Design review of the part built by this model. Coordinates are the model's own, in mm. Face numbers are marked on the shaded views. A direction names the side the tool comes from. Give positions to 0.01 mm unless a question says otherwise; leave off trailing zeros. Loops run counter-clockwise (first coordinate to the right, second up) from the corner with the lowest first, then second, coordinate; pieces in that order, holes last. Notation, with made-up numbers: M 16,40.5 L 66,40.5 A7 cw 66,53.5 Z; hole C 21.5,7.25 d2. An arc over 180 degrees is marked long. Answer as CSV lines item,"result".
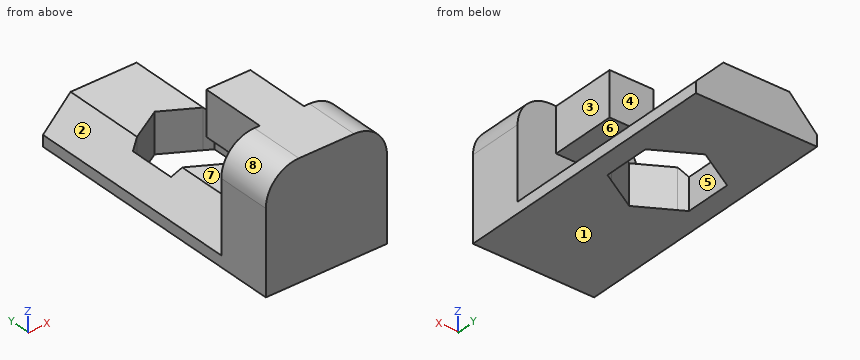
```python
from build123d import *

# Parameters (mm, degrees)
F1_DEPTH = 20
F3_DEPTH = 3.6
F4_W     = 11
F4_H     = 5
F5_DEPTH = 10.5
F6_W     = 4
F6_H     = 4
F7_DEPTH = 6
F8_R     = 3


with BuildPart() as f1:
    # F0 (on Front) → F1 (new body)
    with BuildSketch(Plane.XZ):
        Polygon((-5.5, 0), (5.5, 0), (5.5, 1), (3, 3.6), (0, 3.6), (-3, 3.6), (-5.5, 1), align=None)
    extrude(amount=F1_DEPTH)

    # F2 (on face) → F3 (cut, through all)
    with BuildSketch(Plane.XY.offset(3.6)):
        Polygon((3, -7.459659), (0, -5.727608), (-3, -7.459659), (-3, -12.540341), (0, -14.272392), (3, -12.540341), align=None)
        Polygon((3.7, -7.863804), (3, -7.459659), (3, -12.540341), (3.7, -12.136196), align=None)
        Polygon((-3, -12.540341), (-3, -7.459659), (-3.7, -7.863804), (-3.7, -12.136196), align=None)
    extrude(amount=-F3_DEPTH, mode=Mode.SUBTRACT)

    # F4 (on face) → F5 (join)
    with BuildSketch(Plane(origin=(0, 0, 0), x_dir=(1, 0, 0), z_dir=(0, 0, -1))):
        with Locations((0, 22.5)):
            Rectangle(F4_W, F4_H)
    extrude(amount=-F5_DEPTH)

    # F6 (on face) → F7 (join)
    with BuildSketch(Plane(origin=(0, -20, 0), x_dir=(-1, 0, 0), z_dir=(0, 1, 0))):
        with Locations((0, 8.5)):
            Rectangle(F6_W, F6_H)
    extrude(amount=F7_DEPTH)

    # F8
    f8_edges = [f1.edges().sort_by_distance(p)[0] for p in [
        (-5.5, -22.5, 10.5),
        (5.5, -22.5, 10.5),
    ]]
    fillet(f8_edges, radius=F8_R)


solid = f1.part
```
1. We need section B-B, the plane x = 2.75. Write out the cut boundary in (y, z).
Answer block:
outline,"M -25,0 L -12.68,0 L -12.68,3.6 L -20,3.6 L -20,10.49 L -25,10.49 Z; M -7.32,0 L 0,0 L 0,3.6 L -7.32,3.6 Z"
2. The part is to be moulded in two halves that separate along Z. For the marked faces 5, 6, 7 and 8, say which applies: pulls with the +Z half, pulls with the -Z half, needs draft (parallel to the pull), parting line crosses it, or undercut.
Answer block:
face 5,"needs draft"
face 6,"undercut"
face 7,"undercut"
face 8,"pulls with the +Z half"
3. We need section A-A, the plane y = -16.75. Write out the cut boundary in (x, z).
Answer block:
outline,"M -5.5,0 L 5.5,0 L 5.5,1 L 3,3.6 L -3,3.6 L -5.5,1 Z; M -2,6.5 L 2,6.5 L 2,10.5 L -2,10.5 Z"
4. For P1, Ø1.4, axis at y = -10.5, z = 1.5, coming from the +X side; P2, Ø5, axis at x = -2, z = 8, coming from the +Y side; P3, Ø3, axis at x = -1, y = -2, coming from the +Z side; P4, Ø3, axis at y = -16, z = 9, coming from the +X side, all flat-tipped, find the tip position at first contact; note any pin that passes through.
Answer block:
P1,"x = 5.5"
P2,"y = -14"
P3,"z = 3.6"
P4,"x = 2"
5. To check wall thickness, follow L1, parallel to Z at x = -1, y = -15; L2, parallel to Y at x = -2.5, z = 9.25; L3, parallel to X at y = -16.5, z = 7.5. State the ranges of each line that lie inside material, in increasing order. Write a range as [from, to].
Answer block:
L1,"[0, 3.6], [6.5, 10.5]"
L2,"[-25, -20]"
L3,"[-2, 2]"
6. We need section C-C, the plane z = 7. Write out the cut boundary in (x, y), plus the area to 3 significant figures.
Answer block:
outline,"M -5.5,-25 L 5.5,-25 L 5.5,-20 L 2,-20 L 2,-14 L -2,-14 L -2,-20 L -5.5,-20 Z"
area,"79.0 mm²"
7. For the marked faces 1, 2, 3 and 4, list the 3-axis set-ups (+Z, -Z, +X, -X, +Y, -Y) from which the entire face can be reached by the end or side of a thin tool; tool diameter is ignored.
Answer block:
face 1,"-Z, +X, -X, +Y, -Y"
face 2,"+Z, -X, +Y"
face 3,"+Z, +X, +Y"
face 4,"+Z, +X, -X, +Y"
8. We need section D-D, the plane y = -1.75. Write out the cut boundary in (x, z).
Answer block:
outline,"M -5.5,0 L 5.5,0 L 5.5,1 L 3,3.6 L -3,3.6 L -5.5,1 Z"
